Solid Edge part; units mm, degrees
sketch "Sketch1" plane through (0, 0, 0) normal (0, 0, 1) x (1, 0, 0)
  circle A0 centre (0, 0) radius 9
extrude "Protrusion1" add sketch "Sketch1" along normal mid plane 35
sketch "Sketch2" plane through (0, 0, 0) normal (0, 0, 1) x (1, 0, 0)
  circle A0 centre (0, 0) radius 6
extrude "Cutout1" cut sketch "Sketch2" along normal through all and the other way through all
sketch "Sketch3" plane through (0, 0, 0) normal (0, 0, 1) x (1, 0, 0)
  line L0 (6.3509, 11) -> (-6.3509, 11)
  line L1 (-6.3509, 11) -> (-12.7017, 0)
  line L2 (-12.7017, 0) -> (-6.3509, -11)
  line L3 (-6.3509, -11) -> (6.3509, -11)
  line L4 (6.3509, -11) -> (12.7017, 0)
  line L5 (12.7017, 0) -> (6.3509, 11)
extrude "ExtrudedProtrusion_2" add sketch "Sketch3" along normal mid plane 8
Could you check a few things on this model? Use its own coordinates, in mm. A direction names the side the tool comes from. Round coordinates to 2 decimals unless told otherwise and drop trailing zeros. Loops run counter-clockwise (first coordinate to the right, second up) from the corner with the lowest first, then second, coordinate; pieces in that order, holes last.
Q1. On a 3-axis mill with a long thin cutter (end or side, diameter ignored), from which of +Z, -Z, +X, -X, +Y, -Y can I reach the whole of each face in a straight line? I mean faces 1 (the cylindrical face through (-6, 0, 11)), 2 (the flat face through (9.48, -5.58, -0.06)), 3 (the cylindrical face through (-1.172, 8.923, -10.656)). Say none if no direction works.
Q2. I want a section at C-C (y = -1.5). Write out the boundary of the cut face in (x, z).
Q3. I want a section at A-A (x = 0). Write out the boundary of the cut face in (y, z), and give its area (3 significant figures).
Q4. For P1, Ø3, axis at y = -2, z = -12.5, coming from the +X side; P2, Ø6, axis at y = 5.5, z = 5.5, coming from the -X side; P3, Ø5, axis at y = 8.5, z = 2.5, coming from the -X side; P4, Ø5, axis at x = -5.5, y = 7.5, coming from the -Z side, each with a flat end and sliding along its axis, tell me the tip position at first contact or that it passes through.
Q5. I want a section at B-B (z = 0). Write out the boundary of the cut face in (x, y).
Q6. Please list where these lines run through material, in increasing order: L1, parallel to Y at x = 0, z = 12.25; L2, parallel to Z at x = 6.25, y = -7.5.
Q7. I want a section at D-D (z = 11). Write out the boundary of the cut face in (x, y), and give its area (3 significant figures).
Q8. Thinking about a two-plate mould opening in X: for faces 4 (the flat face through (2, 9, 4)), 5 (the flat face through (0, 0, 4)), 6 (the flat face through (0, 0, -4)), 7 (the cylindrical face through (-1.172, -8.923, 10.656)), which applies, pulls with the +X half, pulls with the -X half, needs draft (parallel to the pull), parting line crosses it, or undercut?
Answer below:
1. face 1: +Z
1. face 2: +Z, -Z, +X, -Y
1. face 3: -Z
2. outline: (-11.84, -4) - (-8.87, -4) - (-8.87, -17.5) - (-5.81, -17.5) - (-5.81, -4) - (5.81, -4) - (5.81, -17.5) - (8.87, -17.5) - (8.87, -4) - (11.84, -4) - (11.84, 4) - (8.87, 4) - (8.87, 17.5) - (5.81, 17.5) - (5.81, 4) - (-5.81, 4) - (-5.81, 17.5) - (-8.87, 17.5) - (-8.87, 4) - (-11.84, 4) - close
3. outline: (-11, -4) - (-9, -4) - (-9, -17.5) - (-6, -17.5) - (-6, -4) - (6, -4) - (6, -17.5) - (9, -17.5) - (9, -4) - (11, -4) - (11, 4) - (9, 4) - (9, 17.5) - (6, 17.5) - (6, 4) - (-6, 4) - (-6, 17.5) - (-9, 17.5) - (-9, 4) - (-11, 4) - close
3. area: 338 mm2
4. P1: stops at x = 8.99
4. P2: stops at x = -11.03
4. P3: stops at x = -9.24
4. P4: stops at z = -17.5
5. outline: (-12.7, 0) - (-6.35, -11) - (6.35, -11) - (12.7, 0) - (6.35, 11) - (-6.35, 11) - close
6. L1: y = -9 to -6, 6 to 9
6. L2: z = -4 to 4
7. outline: circle Ø18 at (0, 0); hole circle Ø12 at (0, 0)
7. area: 141 mm2
8. face 4: needs draft
8. face 5: undercut
8. face 6: undercut
8. face 7: parting line crosses it
